```python
from build123d import *

# Parameters (mm, degrees)
SKETCH1_W                = 20
SKETCH1_H                = 20
BOSS_EXTRUDE1_DEPTH      = 5
BOSS_EXTRUDE2_DEPTH      = 3
BOSS_EXTRUDE2_DEPTH_BACK = 5
SKETCH2_W                = 6
SKETCH2_H                = 27.5
SKETCH2_W_2              = 20
SKETCH2_H_2              = 5
CUT_EXTRUDE1_REACH       = 63.575
SKETCH4_R                = 1.25
SKETCH8_R                = 10.5
CUT_EXTRUDE4_DEPTH       = 5
CUT_EXTRUDE5_REACH       = 66.904
SKETCH9_R                = 9
FILLET2_R                = 1
FILLET3_R                = 2


with BuildPart() as part:
    # Sketch1 → Boss-Extrude1 (new body)
    with BuildSketch(Plane(origin=(0, 0, 0), x_dir=(1, 0, 0), z_dir=(0, 1, 0))):
        with Locations((10, 10)):
            Rectangle(SKETCH1_W, SKETCH1_H)
    extrude(amount=BOSS_EXTRUDE1_DEPTH)

    # Sketch2 → Boss-Extrude2 (add, two sides: drawn at the far end of the back side and taken through both)
    with BuildSketch(Plane(origin=(20, 0, 0), x_dir=(0, 0, -1), z_dir=(1, 0, 0)).offset(-BOSS_EXTRUDE2_DEPTH_BACK)):
        with Locations((17, 18.75)):
            Rectangle(SKETCH2_W, SKETCH2_H)
        with Locations((3, 18.75)):
            Rectangle(SKETCH2_W, SKETCH2_H)
        with Locations((10, 2.5)):
            Rectangle(SKETCH2_W_2, SKETCH2_H_2)
        Polygon((-2.5, 32.5), (0, 32.5), (6, 32.5), (14, 32.5), (20, 32.5), (22.5, 32.5), (22.5, 57.5), (-2.5, 57.5), align=None)
    extrude(amount=BOSS_EXTRUDE2_DEPTH + BOSS_EXTRUDE2_DEPTH_BACK)

    # Sketch4 → Cut-Extrude1 (cut, up to next)
    with BuildSketch(Plane(origin=(0, 5, 0), x_dir=(1, 0, 0), z_dir=(0, 1, 0)), mode=Mode.PRIVATE) as cut_extrude1_sk1:
        with Locations(Location((12, 3, 0), (0, 0, 270))):
            Circle(SKETCH4_R)
    cut_extrude1_tool1 = extrude(cut_extrude1_sk1.sketch, amount=-CUT_EXTRUDE1_REACH, mode=Mode.PRIVATE) & part.part
    # Sketch4 → Cut-Extrude1 (cut, up to next)
    with BuildSketch(Plane(origin=(0, 5, 0), x_dir=(1, 0, 0), z_dir=(0, 1, 0)), mode=Mode.PRIVATE) as cut_extrude1_sk2:
        with Locations(Location((4, 3, 0), (0, 0, 270))):
            Circle(SKETCH4_R)
    cut_extrude1_tool2 = extrude(cut_extrude1_sk2.sketch, amount=-CUT_EXTRUDE1_REACH, mode=Mode.PRIVATE) & part.part
    # Sketch4 → Cut-Extrude1 (cut, up to next)
    with BuildSketch(Plane(origin=(0, 5, 0), x_dir=(1, 0, 0), z_dir=(0, 1, 0)), mode=Mode.PRIVATE) as cut_extrude1_sk3:
        with Locations(Location((12, 17, 0), (0, 0, 90))):
            Circle(SKETCH4_R)
    cut_extrude1_tool3 = extrude(cut_extrude1_sk3.sketch, amount=-CUT_EXTRUDE1_REACH, mode=Mode.PRIVATE) & part.part
    # Sketch4 → Cut-Extrude1 (cut, up to next)
    with BuildSketch(Plane(origin=(0, 5, 0), x_dir=(1, 0, 0), z_dir=(0, 1, 0)), mode=Mode.PRIVATE) as cut_extrude1_sk4:
        with Locations(Location((4, 17, 0), (0, 0, 90))):
            Circle(SKETCH4_R)
    cut_extrude1_tool4 = extrude(cut_extrude1_sk4.sketch, amount=-CUT_EXTRUDE1_REACH, mode=Mode.PRIVATE) & part.part
    add(cut_extrude1_tool1.solids().sort_by_distance((12, 5, -3))[0], mode=Mode.SUBTRACT)
    add(cut_extrude1_tool2.solids().sort_by_distance((4, 5, -3))[0], mode=Mode.SUBTRACT)
    add(cut_extrude1_tool3.solids().sort_by_distance((12, 5, -17))[0], mode=Mode.SUBTRACT)
    add(cut_extrude1_tool4.solids().sort_by_distance((4, 5, -17))[0], mode=Mode.SUBTRACT)

    # Sketch8 → Cut-Extrude4 (cut)
    with BuildSketch(Plane.ZY.offset(-15)):
        with Locations((-10, 45)):
            Circle(SKETCH8_R)
    extrude(amount=-CUT_EXTRUDE4_DEPTH, mode=Mode.SUBTRACT)

    # Sketch9 → Cut-Extrude5 (cut, up to next)
    with BuildSketch(Plane.ZY.offset(-20), mode=Mode.PRIVATE) as cut_extrude5_sk1:
        with Locations((-10, 45)):
            Circle(SKETCH9_R)
    cut_extrude5_tool1 = extrude(cut_extrude5_sk1.sketch, amount=-CUT_EXTRUDE5_REACH, mode=Mode.PRIVATE) & part.part
    add(cut_extrude5_tool1.solids().sort_by_distance((20, 45, -10))[0], mode=Mode.SUBTRACT)

    # Fillet2
    fillet2_edges = [part.edges().sort_by_distance(p)[0] for p in [
        (19, 32.5, -20),
        (19, 32.5, 0),
        (19, 32.5, 2.5),
        (19, 57.5, 2.5),
        (19, 57.5, -22.5),
        (19, 32.5, -22.5),
    ]]
    fillet(fillet2_edges, radius=FILLET2_R)

    # Fillet3
    fillet3_edges = [part.edges().sort_by_distance(p)[0] for p in [
        (19, 5, -6),
        (19, 32.5, -6),
        (19, 5, -14),
        (19, 32.5, -14),
    ]]
    fillet(fillet3_edges, radius=FILLET3_R)


solid = part.part
```
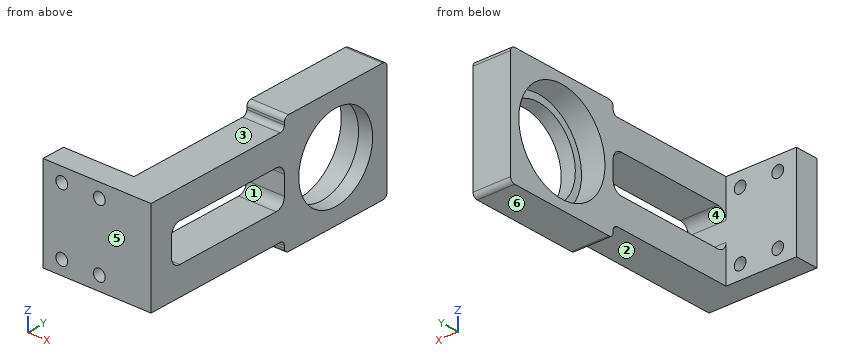
Geometry: final body of the model. Coordinates: model frame, mm. Face numbers are marked on the shaded views. A direction names the side the tool comes from. Round coordinates to 2 decimals unless told otherwise and drop trailing zeros. Loops run counter-clockwise (first coordinate to the right, second up) from the corner with the lowest first, then second, coordinate; pieces in that order, holes last. Notation, with made-up numbers: (41, 66.25) -> (69, 66.25) arc R22 cw to (69, 90.25) -> close; hole circle Ø10 at (-7, 33.25). An arc over 180 degrees is marked (long way). Use one line per item in the form item = value. Start each with the question number.
1) Access query for the marked faces 1, 2 and 3. Directions: +Z, -Z, +X, -X, +Y, -Y. A direction counts if a zero-diameter tool reaches every point of the face in a straight line with its end or side. Return the directions, or none.
2) Section C-C on y = 45. Output: boundary loops of the cut face in (x, z).
3) Section D-D on x = 18.5. Output: boundary loops of the cut face in (y, z), then the cut area to 3 significant figures.
4) Draft query along Y for the marked faces 4, 5 and 6. Return one class per face: released by +Y, released by -Y, zero draft, split by the parting line, or undercut.
5) Section A-A on x = 12. Output: boundary loops of the cut face in (y, z).
6) Line query: L1, parallel to X at y = 1.9, z = -3; L2, parallel to Y at x = 17.5, z = -12.5; L3, parallel to Y at x = 21.5, z = -21. Output: solid intervals per line, ascending.
7) First-contact query: P1, Ø12, axis at x = 4, y = 9, coming from the +Z side; P2, Ø3, axis at x = 4, z = -17, coming from the +Y side; P3, Ø8, axis at y = 37, z = -17, coming from the -X side; P4, Ø4.5, axis at x = 20, z = -9.5, coming from the -Y side. Flat tips, straight axial feed; report the tip coordinate or a pass-through.
8) Section B-B on z = -10. Output: boundary loops of the cut face in (x, y), then the cut area to 3 significant figures.
Response:
q1.face_1 = +X, -X
q1.face_2 = -Z, +X, -X, -Y
q1.face_3 = +Z, +X, -X, -Y
q2.outline = (15, -22.5) -> (23, -22.5) -> (23, -19) -> (20, -19) -> (20, -20.5) -> (15, -20.5) -> close; (15, 0.5) -> (20, 0.5) -> (20, -1) -> (23, -1) -> (23, 2.5) -> (15, 2.5) -> close
q3.outline = (0, -20) -> (31.5, -20) arc R1 cw to (32.5, -21) -> (32.5, -21.5) arc R1 ccw to (33.5, -22.5) -> (56.5, -22.5) arc R1 ccw to (57.5, -21.5) -> (57.5, 1.5) arc R1 ccw to (56.5, 2.5) -> (33.5, 2.5) arc R1 ccw to (32.5, 1.5) -> (32.5, 1) arc R1 cw to (31.5, 0) -> (0, 0) -> close; hole (5, -12) arc R2 ccw to (7, -14) -> (30.5, -14) arc R2 ccw to (32.5, -12) -> (32.5, -8) arc R2 ccw to (30.5, -6) -> (7, -6) arc R2 ccw to (5, -8) -> close; hole circle Ø21 at (45, -10)
q3.area = 712 mm^2
q4.face_4 = undercut
q4.face_5 = released by -Y
q4.face_6 = zero draft
q5.outline = (0, -20) -> (5, -20) -> (5, -18.25) -> (0, -18.25) -> close; (0, -15.75) -> (5, -15.75) -> (5, -4.25) -> (0, -4.25) -> close; (0, -1.75) -> (5, -1.75) -> (5, 0) -> (0, 0) -> close
q6.L1 = 0 to 2.75, 5.25 to 10.75, 13.25 to 23
q6.L2 = 0 to 5.06, 32.44 to 34.8, 55.2 to 57.5
q6.L3 = 32.5 to 57.5
q7.P1 = 0
q7.P2 = 5
q7.P3 = 15
q7.P4 = 0
q8.outline = (0, 0) -> (23, 0) -> (23, 5) -> (0, 5) -> close; (15, 32.5) -> (23, 32.5) -> (23, 36) -> (20, 36) -> (20, 34.5) -> (15, 34.5) -> close; (15, 55.5) -> (20, 55.5) -> (20, 54) -> (23, 54) -> (23, 57.5) -> (15, 57.5) -> close
q8.area = 156 mm^2
